Geometry: final body of the model. Coordinates: model frame, mm. Face numbers are marked on the shaded views. A direction names the side the tool comes from. Give positions to 0.01 mm unless a question says otherwise; leave off trailing zeros. Order: outer loops, then holes, each group sorted by start corner. A loop starts at its lowest first (then second) coordinate and runs counter-clockwise, first axis right, second up. Notation, with made-up numbers: (49.25, -37) - (63.25, -37) arc R17 ccw to (63.25, -20) - close; hole circle Ø1 at (57, 59). An arc over 180 degrees is marked (long way). Write item = value, one per line. Start each with the question number.
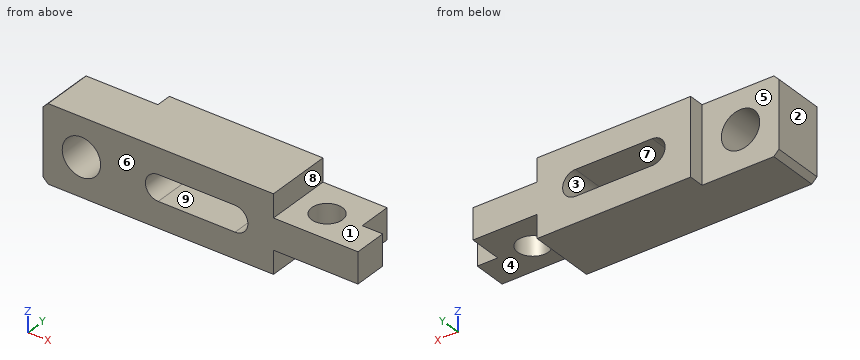
from build123d import *

# Parameters (mm, degrees)
ESTRUSIONE_ESTRUSIONE1_DEPTH = 15
TAGLIO_ESTRUSIONE1_REACH     = 128.61
SCHIZZO5_W                   = 33
SCHIZZO5_H                   = 9
TAGLIO_ESTRUSIONE2_REACH     = 128.61
FORO_15_0_15_2_D             = 15
FORO_12_0_12_2_D             = 12
SMUSSO1_SIZE                 = 2


with BuildPart() as part:
    # Schizzo1 → Estrusione-Estrusione1 (new, symmetric)
    with BuildSketch(Plane.XY):
        Polygon((0, 0), (0, 20), (30, 20), (30, 26), (115, 26), (115, 13), (123, 13), (123, 0), align=None)
    extrude(amount=ESTRUSIONE_ESTRUSIONE1_DEPTH, both=True)

    # Schizzo5 → Taglio-Estrusione1 (cut, up to next)
    with BuildSketch(Plane(origin=(0, 26, 0), x_dir=(1, 0, 0), z_dir=(0, 1, 0)), mode=Mode.PRIVATE) as taglio_estrusione1_sk1:
        with Locations((106.5, 10.5)):
            Rectangle(SCHIZZO5_W, SCHIZZO5_H)
    taglio_estrusione1_tool1 = extrude(taglio_estrusione1_sk1.sketch, amount=-TAGLIO_ESTRUSIONE1_REACH, mode=Mode.PRIVATE) & part.part
    # Schizzo5 → Taglio-Estrusione1 (cut, up to next)
    with BuildSketch(Plane(origin=(0, 26, 0), x_dir=(1, 0, 0), z_dir=(0, 1, 0)), mode=Mode.PRIVATE) as taglio_estrusione1_sk2:
        with Locations((106.5, -10.5)):
            Rectangle(SCHIZZO5_W, SCHIZZO5_H)
    taglio_estrusione1_tool2 = extrude(taglio_estrusione1_sk2.sketch, amount=-TAGLIO_ESTRUSIONE1_REACH, mode=Mode.PRIVATE) & part.part
    add(taglio_estrusione1_tool1.solids().sort_by_distance((106.5, 26, -10.5))[0], mode=Mode.SUBTRACT)
    add(taglio_estrusione1_tool2.solids().sort_by_distance((106.5, 26, 10.5))[0], mode=Mode.SUBTRACT)

    # Schizzo6 → Taglio-Estrusione2 (cut, up to next)
    with BuildSketch(Plane(origin=(0, 26, 0), x_dir=(1, 0, 0), z_dir=(0, 1, 0)), mode=Mode.PRIVATE) as taglio_estrusione2_sk1:
        with BuildLine():
            Line((45, 5), (75, 5))
            ThreePointArc((75, 5), (80, 0), (75, -5))
            Line((75, -5), (45, -5))
            ThreePointArc((45, -5), (40, 0), (45, 5))
        make_face()
    taglio_estrusione2_tool1 = extrude(taglio_estrusione2_sk1.sketch, amount=-TAGLIO_ESTRUSIONE2_REACH, mode=Mode.PRIVATE) & part.part
    add(taglio_estrusione2_tool1.solids().sort_by_distance((60, 26, 0))[0], mode=Mode.SUBTRACT)

    # Foro Ø15.0 (15)-2 (through all)
    with Locations(Plane(origin=(15, 20, 0), x_dir=(0, 0, 1), z_dir=(0, 1, 0))):
        with Locations((0, 0)):
            Hole(FORO_15_0_15_2_D / 2)

    # Foro Ø12.0 (12)-2 (through all)
    with Locations(Plane(origin=(102, 12, 6), x_dir=(1, 0, 0), z_dir=(0, 0, 1))):
        with Locations((0, 0)):
            Hole(FORO_12_0_12_2_D / 2)

    # Smusso1
    smusso1_edges = [part.edges().sort_by_distance(p)[0] for p in [
        (0, 10, -15),
        (0, 10, 15),
    ]]
    chamfer(smusso1_edges, length=SMUSSO1_SIZE)


solid = part.part
Q1. Set-up query: the marked faces 1, 2, 3, 4 and 5. Return all of +Z, -Z, +X, -X, +Y, -Y with unobstructed straight access to the full face (end or side cutting, diameter ignored); none if empty.
Q2. Material intervals for line 1 along X through (y, z) = (8.25, 0); line 2 along Y through (x, z) = (102, 1.25); line 3 along X through (y, z) = (9, 3), sorted ascending. Write a range as from..to.
Q3. Pull-direction query (X, two-part tool) for the marked faces 6, 7, 8 and 9; classes: +X half, -X half, draft (parallel to the pull), parting line (faces both ways), or undercut.
Q4. Section B-B, the plane x = 102. Return the cut outline in (y, z).
Q5. Section C-C, the plane y = 9. Return the cut outline in (x, z).
Q6. Contact query for flat-ended pins moving along their axis: pin 1 (1.5 mm diameter, centred on x = 108.5, z = -7.5, fed in from -Y); pin 2 (13 mm diameter, centred on x = 99, y = 17.5, fed in from +Z); pin 3 (4.5 mm diameter, centred on y = 17, z = -9, fed in from +X); pin 4 (9 mm diameter, centred on x = 21, z = -7, fed in from +Y). Output: stop coordinate, or through.
Q7. Section A-A, the plane z = 0. Return the cut outline in (x, y), then the cut area to 3 significant figures.
Q8. Section D-D, the plane x = 15. Return the cut outline in (y, z).
The answers:
q1.face_1 = +Z, +X, +Y, -Y
q1.face_2 = +Z, -Z, -X, +Y, -Y
q1.face_3 = +Y, -Y
q1.face_4 = -Z, +X, +Y, -Y
q1.face_5 = +Z, -Z, -X, +Y
q2.line_1 = 0..7.5, 22.5..40, 80..97.32, 106.68..123
q2.line_2 = 0..6, 18..26
q2.line_3 = 0..8.13, 21.87..41, 79..96.8, 107.2..123
q3.face_6 = draft
q3.face_7 = undercut
q3.face_8 = +X half
q3.face_9 = undercut
q4.outline = (0, -6) - (6, -6) - (6, 6) - (0, 6) - close; (18, -6) - (26, -6) - (26, 6) - (18, 6) - close
q5.outline = (0, -13) - (2, -15) - (90, -15) - (90, -6) - (96.8, -6) - (96.8, 6) - (90, 6) - (90, 15) - (2, 15) - (0, 13) - close; (107.2, -6) - (123, -6) - (123, 6) - (107.2, 6) - close; hole circle Ø15 at (15, 0); hole (45, -5) - (75, -5) arc R5 ccw to (75, 5) - (45, 5) arc R5 ccw to start
q6.pin_1 = through
q6.pin_2 = 6
q6.pin_3 = 90
q6.pin_4 = 20
q7.outline = (0, 0) - (7.5, 0) - (7.5, 20) - (0, 20) - close; (22.5, 0) - (40, 0) - (40, 26) - (30, 26) - (30, 20) - (22.5, 20) - close; (80, 0) - (123, 0) - (123, 13) - (115, 13) - (115, 26) - (80, 26) - close; hole circle Ø12 at (102, 12)
q7.area = 1,460 mm²
q8.outline = (0, -15) - (20, -15) - (20, -7.5) - (0, -7.5) - close; (0, 7.5) - (20, 7.5) - (20, 15) - (0, 15) - close
